Build history of the part. All positions in model axes, mm. A direction names the side the tool comes from. Give positions to 0.01 mm unless a question says otherwise; leave off trailing zeros. Write each loop counter-clockwise with the first axis right and the second up, starting at its lowest first coordinate (ties: lowest second). Pieces come first, ordered by that corner, then holes. Notation, with made-up numbers: (-38.75, 74) -> (-15.75, 74) arc R19 ccw to (-15.75, 92) -> close; hole circle Ø4 at (71, -29). An arc over 180 degrees is marked (long way). Put each result on its own line as item: value. Start each with the question number.
Item 1: Slice it at A-A, the plane x = 0. List the corners of the cut face in (y, z), plus the area to 3 significant figures.
Item 2: Two-plate mould, pull along Z, no slides. Class faces 3 (the cylindrical face through (-21, 3, -28)), 4 (the flat face through (-15, 0, 0)), 5 (the cylindrical face through (5.497, 4.2, 14.943)): pulls with the +Z half, pulls with the -Z half, needs draft (parallel to the pull), parting line crosses it, or undercut.
Item 3: Slice it at B-B, the plane z = 0. List the corners of the cut face in (x, y), plus the area to 3 significant figures.
Item 4: Slice it at D-D, the plane y = 3.25. List the corners of the cut face in (x, z), plus the area to 3 significant figures.
Item 5: Flat gauge pins, fed straight in: pin 1 Ø2 at (y, z) = (6, 12.5) entering from -X; pin 2 Ø1.5 at (x, y) = (-2.5, 2.5) entering from -Z; pin 3 Ø5 at (x, z) = (-15.33, 0) entering from +Y; pin 4 Ø22.5 at (x, z) = (0, 0) entering from +Y. Where does each tip first touch, or does it go through?
Item 6: Slice it at C-C, the plane x = -11. List the corners of the cut face in (y, z).
Item 7: Drill centre lines: line 1 along Z through (x, y) = (7.5, 6.5); line 2 along Z through (x, y) = (8, 2.25); line 3 along Z through (x, y) = (-8, 1.75). Where is each one in solid material? Low to high.
Item 8: Tool access for faces 1 (the cylindrical face through (3.755, 3.451, 11.923)), 2 (the flat face through (-15, 1.477, 0)): list every direction of +Z, -Z, +X, -X, +Y, -Y with a clear straight run to the whole face (end or side of a thin tool).
```python
from build123d import *

# Parameters (mm, degrees)
SKETCH1_R             = 35
BOSS_EXTRUDE1_DEPTH   = 7
SKETCH2_R             = 12.5
CUT_EXTRUDE1_DEPTH    = 50.989999
SKETCH3_R             = 2.734497858
CUT_EXTRUDE2_DEPTH    = 5.523438
CIRPATTERN1_START     = 1.476561887
CIRPATTERN1_OUTLINE_R = 2.734497858
CIRPATTERN1_DEPTH     = 5.523438113


# Read off the part's stored shape, not the designer's step: CirPattern1
with BuildPart() as part:
    # Sketch1 → Boss-Extrude1 (new body)
    with BuildSketch(Plane(origin=(0, 0, 0), x_dir=(1, 0, 0), z_dir=(0, 1, 0))):
        with Locations(Location((0, 0, 0), (0, 0, 270))):
            Circle(SKETCH1_R)
    extrude(amount=BOSS_EXTRUDE1_DEPTH)

    # Sketch2 → Cut-Extrude1 (cut, through all)
    with BuildSketch(Plane(origin=(0, 0, 0), x_dir=(1, 0, 0), z_dir=(0, 1, 0))):
        with Locations(Location((0, 0, 0), (0, 0, 270))):
            Circle(SKETCH2_R)
    extrude(amount=CUT_EXTRUDE1_DEPTH, mode=Mode.SUBTRACT)

    # Sketch3 → Cut-Extrude2 (cut)
    with BuildSketch(Plane(origin=(0, 7, 0), x_dir=(1, 0, 0), z_dir=(0, 1, 0))):
        with Locations(Location((-15.333559702, 0, 0), (0, 0, 270))):
            Circle(SKETCH3_R)
    extrude(amount=-CUT_EXTRUDE2_DEPTH, mode=Mode.SUBTRACT)

    # CirPattern1 outline → CirPattern1 (cut)
    with BuildSketch(Plane(origin=(0, 0, 0), x_dir=(1, 0, 0), z_dir=(0, 1, 0)).offset(CIRPATTERN1_START)):
        with Locations((7.666779851, 13.279252232)):
            Circle(CIRPATTERN1_OUTLINE_R)
        with Locations((7.666779851, -13.279252232)):
            Circle(CIRPATTERN1_OUTLINE_R)
    extrude(amount=CIRPATTERN1_DEPTH, mode=Mode.SUBTRACT)


solid = part.part
```
Values follow:
1. outline: (0, -35) -> (7, -35) -> (7, -12.5) -> (0, -12.5) -> close; (0, 12.5) -> (7, 12.5) -> (7, 35) -> (0, 35) -> close
1. area: 315 mm2
2. face 3: parting line crosses it
2. face 4: needs draft
2. face 5: undercut
3. outline: (-35, 0) -> (-12.5, 0) -> (-12.5, 7) -> (-12.6, 7) -> (-12.6, 1.48) -> (-18.07, 1.48) -> (-18.07, 7) -> (-35, 7) -> close; (12.5, 0) -> (35, 0) -> (35, 7) -> (12.5, 7) -> close
3. area: 285 mm2
4. outline: circle Ø70 at (0, 0); hole circle Ø5.47 at (-15.33, 0); hole circle Ø25 at (0, 0); hole circle Ø5.47 at (7.67, -13.28); hole circle Ø5.47 at (7.67, 13.28)
4. area: 3,290 mm2
5. pin 1: x = -33.06
5. pin 2: z = -34.96
5. pin 3: y = 1.48
5. pin 4: through
6. outline: (0, -33.23) -> (7, -33.23) -> (7, -5.94) -> (0, -5.94) -> close; (0, 5.94) -> (7, 5.94) -> (7, 33.23) -> (0, 33.23) -> close
7. line 1: -34.19 to -16.01, -10.55 to -10, 10 to 10.55, 16.01 to 34.19
7. line 2: -34.07 to -15.99, -10.57 to -9.6, 9.6 to 10.57, 15.99 to 34.07
7. line 3: -34.07 to -9.6, 9.6 to 34.07
8. face 1: +Y, -Y
8. face 2: +Y
